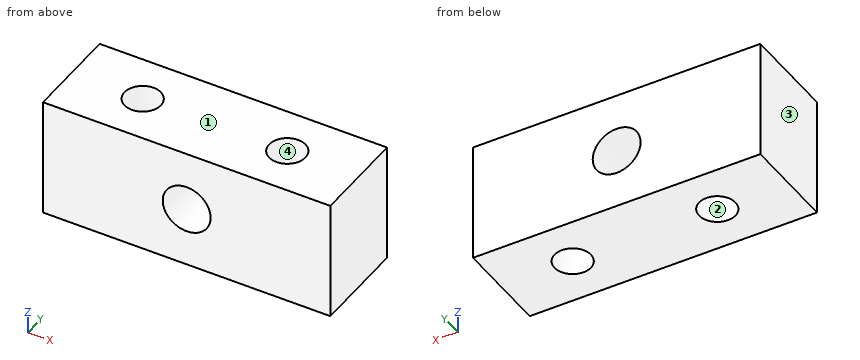
from build123d import *

# Parameters (mm, degrees)
SKETCH1_W           = 38.1
SKETCH1_H           = 15.875
BOSS_EXTRUDE1_DEPTH = 12.7
SKETCH2_R           = 2.413
CUT_EXTRUDE1_DEPTH  = 16.875
SKETCH3_R           = 3.175
CUT_EXTRUDE2_DEPTH  = 13.7


with BuildPart() as part:
    # Sketch1 → Boss-Extrude1 (new body)
    with BuildSketch(Plane(origin=(0, 0, 0), x_dir=(1, 0, 0), z_dir=(0, 1, 0))):
        Rectangle(SKETCH1_W, SKETCH1_H)
    extrude(amount=BOSS_EXTRUDE1_DEPTH)

    # Sketch2 → Cut-Extrude1 (cut, through all)
    with BuildSketch(Plane(origin=(0, 0, -7.9375), x_dir=(-1, 0, 0), z_dir=(0, 0, -1))):
        with Locations((-9.5885, 6.35)):
            Circle(SKETCH2_R)
        with Locations((9.5885, 6.35)):
            Circle(SKETCH2_R)
    extrude(amount=-CUT_EXTRUDE1_DEPTH, mode=Mode.SUBTRACT)

    # Sketch3 → Cut-Extrude2 (cut, through all)
    with BuildSketch(Plane(origin=(0, 12.7, 0), x_dir=(1, 0, 0), z_dir=(0, 1, 0))):
        Circle(SKETCH3_R)
    extrude(amount=-CUT_EXTRUDE2_DEPTH, mode=Mode.SUBTRACT)


solid = part.part
The model under review builds one solid part; all positions refer to its coordinate system, in mm. Face numbers are marked on the shaded views. Give positions to 0.01 mm unless a question says otherwise; leave off trailing zeros. Loops run counter-clockwise (first coordinate to the right, second up) from the corner with the lowest first, then second, coordinate; pieces in that order, holes last. Notation, with made-up numbers: (59.5, 4.5) -> (88.5, 4.5) arc R9 ccw to (88.5, 12.5) -> close; hole circle Ø9 at (54.5, -33). An arc over 180 degrees is marked (long way). Answer as a JSON object with one key per item and string values. Group by question number.
Q1. Draft analysis for pull direction X (two halves, no side actions). For the marked faces 1, 2, 3 and 4, state which applies: pulls with the +X half, pulls with the -X half, needs draft (parallel to the pull), parting line crosses it, or undercut.
Q2. Take a section at D-D (z = 6.5). Write out the cut boundary in (x, y).
Q3. Take a section at A-A (y = 6.35). State how many separate pieces and enclosed holes the cut face has, plus the area to 3 significant figures.
Q4. Take a section at B-B (z = -1.75). Write out the cut boundary in (x, y).
Q5. Wall thickness on line 1 along X through (y, z) = (7.25, -4.25); line 2 along X through (y, z) = (7.5, 6); line 3 along X through (y, z) = (9, 0) (3 decimals): over which ranges is each line inside the solid? List them lowest first.
Q6. Take a section at C-C (x = 0). Write out the cut boundary in (y, z) (1 decimal), plus the area to 3 significant figures.
Answer below:
{
 "1": {"face 1": "needs draft", "face 2": "undercut", "face 3": "pulls with the -X half", "face 4": "undercut"},
 "2": {"outline": "(-19.05, 0) -> (19.05, 0) -> (19.05, 12.7) -> (-19.05, 12.7) -> close; hole circle Ø4.83 at (-9.59, 6.35); hole circle Ø4.83 at (9.59, 6.35)"},
 "3": {"separate pieces": "3", "enclosed holes": "1", "area": "420 mm2"},
 "4": {"outline": "(-19.05, 0) -> (-2.65, 0) -> (-2.65, 12.7) -> (-19.05, 12.7) -> close; (2.65, 0) -> (19.05, 0) -> (19.05, 12.7) -> (2.65, 12.7) -> close; hole circle Ø4.83 at (-9.59, 6.35); hole circle Ø4.83 at (9.59, 6.35)"},
 "5": {"line 1": "x = -19.05 to -11.83, -7.35 to 7.35, 11.83 to 19.05", "line 2": "x = -19.05 to -11.71, -7.47 to 7.47, 11.71 to 19.05", "line 3": "x = -19.05 to -3.175, 3.175 to 19.05"},
 "6": {"outline": "(0, -7.9) -> (12.7, -7.9) -> (12.7, -3.2) -> (0, -3.2) -> close; (0, 3.2) -> (12.7, 3.2) -> (12.7, 7.9) -> (0, 7.9) -> close", "area": "121 mm2"}
}
